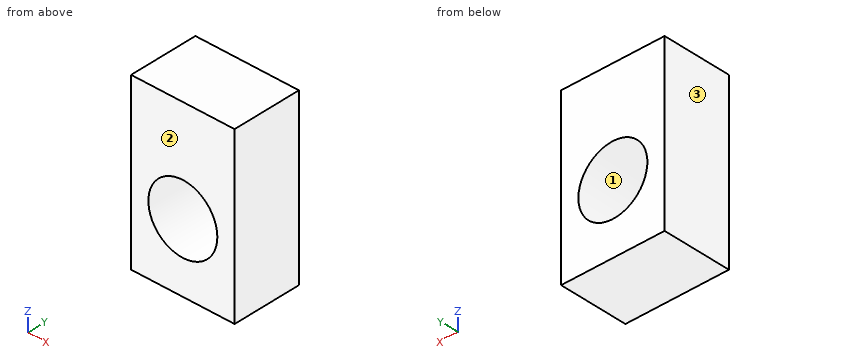
```python
from build123d import *

# Parameters (mm, degrees)
SKETCH1_W           = 30
SKETCH1_H           = 50
SKETCH1_R           = 10
BOSS_EXTRUDE1_DEPTH = 10


with BuildPart() as part:
    # Sketch1 → Boss-Extrude1 (new body, symmetric)
    with BuildSketch(Plane(origin=(0, 0, 0), x_dir=(1, 0, 0), z_dir=(0, 1, 0))):
        with Locations((15, 25)):
            Rectangle(SKETCH1_W, SKETCH1_H)
        with Locations((15, 30)):
            Circle(SKETCH1_R, mode=Mode.SUBTRACT)
    extrude(amount=BOSS_EXTRUDE1_DEPTH, both=True)


solid = part.part
```
Here's how the part is built. I have some questions about the finished solid (model axes, mm). Face numbers are marked on the shaded views. Give positions to 0.01 mm unless a question says otherwise; leave off trailing zeros. Loops run counter-clockwise (first coordinate to the right, second up) from the corner with the lowest first, then second, coordinate; pieces in that order, holes last. Notation, with made-up numbers: M -8,13 L 46,13 A26 cw 46,42 Z; hole C -8.5,84.25 d6. An arc over 180 degrees is marked long. Put each result on its own line as item: value. Start each with the question number.
(1) If we mould it in two halves opening along X, with no side actions, what happens to the marked faces 1, 2 and 3? For each: +X half, -X half, draft (parallel to the pull), parting line (faces both ways), or undercut.
(2) Will this pin go through, and if not, where does the flat tip stop? pin 1 Ø16 at (x, z) = (15, -30) entering from -Y.
(3) I want a section at C-C on y = -2. Please give me the cut outline in (x, z).
(4) I want a section at A-A on z = -30. Please give me the cut outline in (x, y).
(5) I want a section at B-B on x = 15. Please give me the cut outline in (y, z).
(6) I need wall thicknesses on line 1 along Z through (x, y) = (15, -2.5); line 2 along X through (y, z) = (0.75, -30); line 3 along Z through (x, y) = (11.5, -0.25). Which ranges of each line are inside material? Lowest first, please. Write a range as [from, to].
Answer block:
1. face 1: undercut
1. face 2: draft
1. face 3: -X half
2. pin 1: through
3. outline: M 0,-50 L 30,-50 L 30,0 L 0,0 Z; hole C 15,-30 d20
4. outline: M 0,-10 L 5,-10 L 5,10 L 0,10 Z; M 25,-10 L 30,-10 L 30,10 L 25,10 Z
5. outline: M -10,-50 L 10,-50 L 10,-40 L -10,-40 Z; M -10,-20 L 10,-20 L 10,0 L -10,0 Z
6. line 1: [-50, -40], [-20, 0]
6. line 2: [0, 5], [25, 30]
6. line 3: [-50, -39.37], [-20.63, 0]
